Could you check a few things on this drawing? It's one solid part, dimensions in mm from its lowest x, y, z. Round coordinates to 2 decimals unless told otherwise and drop trailing zeros. Write each loop counter-clockwise with the first axis right and the second up, starting at its lowest first coordinate (ties: lowest second). Pieces come first, ordered by that corner, then holes. Notation, with made-up numbers: (77.5, 31.25) -> (93.5, 31.25) arc R13 ccw to (93.5, 35.25) -> close; hole circle Ø8 at (10.25, 81). An arc over 180 degrees is marked (long way). Put each result on its own line as item: value. Start each with the question number.
1) If I drill on line 1 along Y through (x, z) = (10, 3.5); line 2 along Y through (x, z) = (80, 9.75); line 3 along X through (y, z) = (51.5, 8.25), over which ranges is the centre line in solid material (lowest first)? Write a range as [from, to].
2) I want a section at A-A, the plane x = 10. List the corners of the cut face in (y, z) for me.
3) I want a section at B-B, the plane y = 19.5. List the corners of the cut face in (x, z) for me, then the cut area to 3 significant figures.
4) Will these pins go through, and if not, where does the flat tip stop? P1, Ø11, axis at x = 66, z = 3.5, coming from the -Y side; P2, Ø1.5, axis at y = 34.5, z = 14, coming from the +X side; P3, Ø19, axis at x = 10, y = 32.5, coming from the +Z side.
5) I want a section at D-D, the plane x = 130. List the corners of the cut face in (y, z) for me, then the cut area to 3 significant figures.
6) We'd pull the mould along Y, two halves only. Please class the marked faces 1, 2 and 3: released by +Y, released by -Y, zero draft, split by the parting line, or undercut.
7) I want a section at C-C, the plane z = 3. List the corners of the cut face in (x, y) for me.
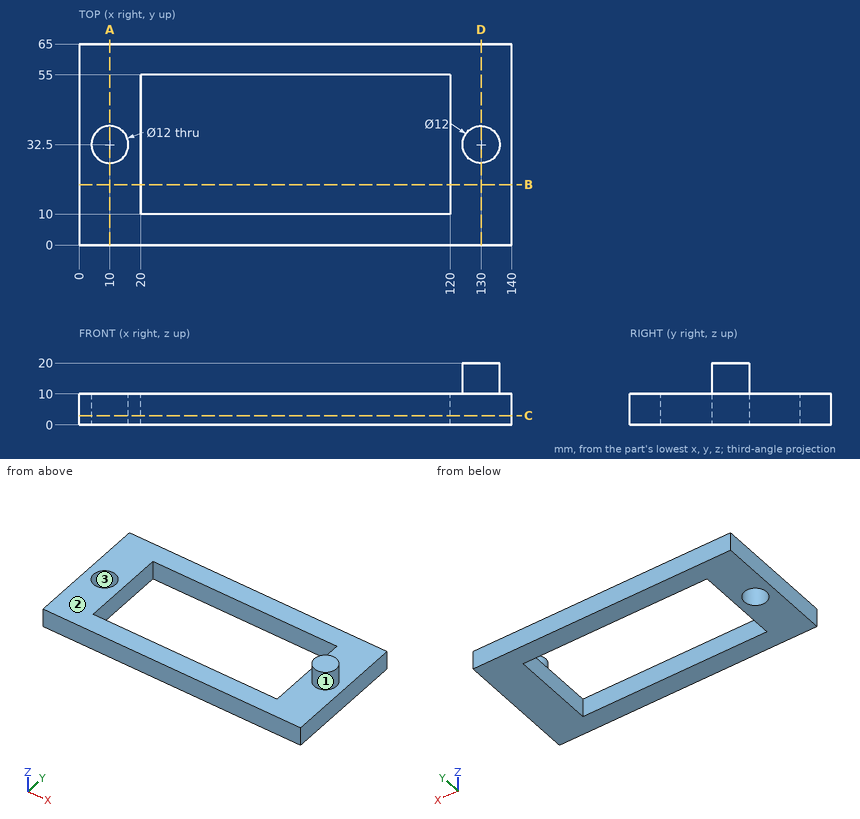
Findings:
1. line 1: y = [0, 26.5], [38.5, 65]
1. line 2: y = [0, 10], [55, 65]
1. line 3: x = [0, 20], [120, 140]
2. outline: (0, 0) -> (26.5, 0) -> (26.5, 10) -> (0, 10) -> close; (38.5, 0) -> (65, 0) -> (65, 10) -> (38.5, 10) -> close
3. outline: (0, 0) -> (20, 0) -> (20, 10) -> (0, 10) -> close; (120, 0) -> (140, 0) -> (140, 10) -> (120, 10) -> close
3. area: 400 mm2
4. P1: stops at y = 0
4. P2: stops at x = 135.87
4. P3: stops at z = 10
5. outline: (0, 0) -> (65, 0) -> (65, 10) -> (38.5, 10) -> (38.5, 20) -> (26.5, 20) -> (26.5, 10) -> (0, 10) -> close
5. area: 770 mm2
6. face 1: split by the parting line
6. face 2: zero draft
6. face 3: undercut
7. outline: (0, 0) -> (140, 0) -> (140, 65) -> (0, 65) -> close; hole circle Ø12 at (10, 32.5); hole (20, 10) -> (120, 10) -> (120, 55) -> (20, 55) -> close
